```python
from build123d import *

# Parameters (mm, degrees)
SKETCH1_W           = 50.8
SKETCH1_H           = 50.8
BOSS_EXTRUDE1_DEPTH = 2.54
SKETCH2_W           = 7.62
SKETCH2_H           = 15.24
BOSS_EXTRUDE2_DEPTH = 104.14
SKETCH3_W           = 12.7
SKETCH3_H           = 22.86
CUT_EXTRUDE1_DEPTH  = 114.485710554


with BuildPart() as part:
    # Sketch1 → Boss-Extrude1 (new body)
    with BuildSketch(Plane(origin=(0, 0, 0), x_dir=(1, 0, 0), z_dir=(0, 1, 0))):
        Rectangle(SKETCH1_W, SKETCH1_H)
    extrude(amount=BOSS_EXTRUDE1_DEPTH)

    # Sketch2 → Boss-Extrude2 (add)
    with BuildSketch(Plane(origin=(0, 2.54, 0), x_dir=(1, 0, 0), z_dir=(0, 1, 0))):
        with Locations((0, 15.24)):
            Rectangle(SKETCH2_W, SKETCH2_H)
    extrude(amount=BOSS_EXTRUDE2_DEPTH)

    # Sketch3 → Cut-Extrude1 (cut, through all)
    with BuildSketch(Plane.ZY.offset(3.81)):
        with Locations((-15.24, 87.63)):
            Rectangle(SKETCH3_W, SKETCH3_H)
    extrude(amount=-CUT_EXTRUDE1_DEPTH, mode=Mode.SUBTRACT)


solid = part.part
```
Can you work these out from the model? Positions are in its coordinate system, mm. A direction names the side the tool comes from. Coordinates: 2 decimals unless noted, no trailing zeros. Write each loop counter-clockwise with the first axis right and the second up, starting at its lowest first coordinate (ties: lowest second). Pieces come first, ordered by that corner, then holes. Notation, with made-up numbers: (24, 62) - (76, 62) arc R32 cw to (76, 100) - close; hole circle Ø2 at (-10.5, -31). An arc over 180 degrees is marked (long way). Return JSON: item names as keys, results as strings.
Q1. Please list where these lines run through material, in increasing order: L1, parallel to Y at x = 1, z = -19.5; L2, parallel to Z at x = 0, y = 68.5; L3, parallel to Y at x = -12.5, z = 7. Write a range as from..to.
Computed values:
{"L1": "y = 0..76.2, 99.06..106.68", "L2": "z = -22.86..-7.62", "L3": "y = 0..2.54"}
Q2. If we section it at C-C (x = 15): Please give me the cut outline in (y, z), then the cut area to 3 significant figures.
Computed values:
{"outline": "(0, -25.4) - (2.54, -25.4) - (2.54, 25.4) - (0, 25.4) - close", "area": "129 mm2"}
Q3. If we section it at B-B (x = -2.5): Please give me the cut outline in (y, z).
Computed values:
{"outline": "(0, -25.4) - (2.54, -25.4) - (2.54, -22.86) - (106.68, -22.86) - (106.68, -7.62) - (2.54, -7.62) - (2.54, 25.4) - (0, 25.4) - close; hole (76.2, -21.59) - (99.06, -21.59) - (99.06, -8.89) - (76.2, -8.89) - close"}
Q4. Thinking about a two-plate mould opening in Y: for faces 1 (the flat face through (0, 87, -8.89)), 2 (the flat face through (0, 1, 25.4)), 3 (the flat face through (0, 106.68, -15)), which applies, +Y half, -Y half, draft (parallel to the pull), parting line (faces both ways), or undercut?
Computed values:
{"face 1": "undercut", "face 2": "draft", "face 3": "+Y half"}
Q5. If we section it at D-D (z = -6.5): Please give me the cut outline in (x, y), then the cut area to 3 significant figures.
Computed values:
{"outline": "(-25.4, 0) - (25.4, 0) - (25.4, 2.54) - (-25.4, 2.54) - close", "area": "129 mm2"}
Q6. On a 3-axis mill with a long thin cutter (end or side, diameter ignored), from which of +Z, -Z, +X, -X, +Y, -Y can I reach the whole of each face in a straight line? I mean faces 4 (the flat face through (-3.81, 42, -15)), 5 (the flat face through (0, 87, -21.59)), 6 (the flat face through (0, 54, -7.62)). Say none if no direction works.
Computed values:
{"face 4": "+Z, -Z, -X, +Y", "face 5": "+X, -X", "face 6": "+Z, +X, -X, +Y"}
Q7. I'm going to push flat-ended pins straight in: pin 1 Ø5 at (x, z) = (-8, -5) entering from -Y; pin 2 Ø12 at (y, z) = (71, -15) entering from -X; pin 3 Ø15 at (x, z) = (11.5, 4.5) entering from +Y; pin 4 Ø4 at (x, y) = (0, 47.5) entering from -Z. Where does each tip first touch, or does it pass through?
Computed values:
{"pin 1": "stops at y = 0", "pin 2": "stops at x = -3.81", "pin 3": "stops at y = 2.54", "pin 4": "stops at z = -22.86"}
Q8. If we section it at A-A (z = -17): Please give me the cut outline in (x, y).
Computed values:
{"outline": "(-25.4, 0) - (25.4, 0) - (25.4, 2.54) - (3.81, 2.54) - (3.81, 76.2) - (-3.81, 76.2) - (-3.81, 2.54) - (-25.4, 2.54) - close; (-3.81, 99.06) - (3.81, 99.06) - (3.81, 106.68) - (-3.81, 106.68) - close"}
